Design review of the part built by this model. Coordinates are the model's own, in mm. Face numbers are marked on the shaded views. A direction names the side the tool comes from. Give positions to 0.01 mm unless a question says otherwise; leave off trailing zeros. Write each loop counter-clockwise with the first axis right and the second up, starting at its lowest first coordinate (ties: lowest second). Pieces come first, ordered by that corner, then holes. Notation, with made-up numbers: (17, 3.25) -> (38, 3.25) arc R6 cw to (38, 10.25) -> close; hole circle Ø5 at (47.25, 47). An arc over 180 degrees is marked (long way). Answer as a JSON object with one key per item and string values.
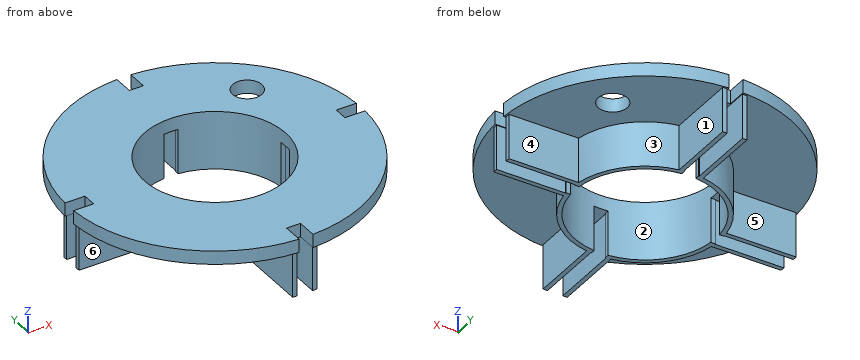
```python
from build123d import *

# Parameters (mm, degrees)
CYLINDER_R     = 3.25
CYLINDER_DEPTH = 10
BOX030_W       = 3
BOX030_H       = 3
BOX030_DEPTH   = 3
BOX047_W       = 3
BOX047_H       = 3
BOX047_DEPTH   = 3
BOX029_W       = 3
BOX029_H       = 3
BOX029_DEPTH   = 3
BOX028_W       = 3
BOX028_H       = 3
BOX028_DEPTH   = 3
BOX043_W       = 3.1
BOX043_H       = 6
BOX043_DEPTH   = 10
BOX044_W       = 3.1
BOX044_H       = 6
BOX044_DEPTH   = 10
BOX045_W       = 6
BOX045_H       = 3.1
BOX045_DEPTH   = 10
BOX046_W       = 6
BOX046_H       = 3.1
BOX046_DEPTH   = 10
BOX032_W       = 3.1
BOX032_H       = 6
BOX032_DEPTH   = 3
BOX033_W       = 6
BOX033_H       = 3.1
BOX033_DEPTH   = 3
BOX034_W       = 6
BOX034_H       = 3.1
BOX034_DEPTH   = 3
BOX031_W       = 3.1
BOX031_H       = 6
BOX031_DEPTH   = 3
TUBE003_R      = 16.7
TUBE003_R_2    = 15.7
TUBE003_DEPTH  = 10
BOX036_W       = 1
BOX036_H       = 16
BOX036_DEPTH   = 10
BOX037_W       = 1
BOX037_H       = 16
BOX037_DEPTH   = 10
BOX038_W       = 1
BOX038_H       = 16
BOX038_DEPTH   = 10
BOX039_W       = 16
BOX039_H       = 1
BOX039_DEPTH   = 10
BOX040_W       = 16
BOX040_H       = 1
BOX040_DEPTH   = 10
BOX041_W       = 16
BOX041_H       = 1
BOX041_DEPTH   = 10
BOX042_W       = 16
BOX042_H       = 1
BOX042_DEPTH   = 10
BOX035_W       = 1
BOX035_H       = 16
BOX035_DEPTH   = 10
TUBE002_R      = 32.5
TUBE002_R_2    = 15.7
TUBE002_DEPTH  = 3


with BuildPart() as eyeboltcutout:
    # Cylinder → Cylinder (new body)
    with BuildSketch(Plane(origin=(17.5, 16.5, 91), x_dir=(1, 0, 0), z_dir=(0, 0, 1))):
        Circle(CYLINDER_R)
    extrude(amount=CYLINDER_DEPTH)


with BuildPart() as finlock015:
    # Box030 → Box030 (new body)
    with BuildSketch(Plane(origin=(-1.5, 21, -3), x_dir=(1, 0, 0), z_dir=(0, 0, 1))):
        with Locations((1.5, 1.5)):
            Rectangle(BOX030_W, BOX030_H)
    extrude(amount=BOX030_DEPTH)


with BuildPart() as finlock016:
    # Box047 → Box047 (new body)
    with BuildSketch(Plane(origin=(-1.5, -24, -3), x_dir=(1, 0, 0), z_dir=(0, 0, 1))):
        with Locations((1.5, 1.5)):
            Rectangle(BOX047_W, BOX047_H)
    extrude(amount=BOX047_DEPTH)


with BuildPart() as finlock014:
    # Box029 → Box029 (new body)
    with BuildSketch(Plane(origin=(-24, -1.5, -3), x_dir=(1, 0, 0), z_dir=(0, 0, 1))):
        with Locations((1.5, 1.5)):
            Rectangle(BOX029_W, BOX029_H)
    extrude(amount=BOX029_DEPTH)


with BuildPart() as finlocks001:
    # Box028 → Box028 (new body)
    with BuildSketch(Plane(origin=(21, -1.5, -3), x_dir=(1, 0, 0), z_dir=(0, 0, 1))):
        with Locations((1.5, 1.5)):
            Rectangle(BOX028_W, BOX028_H)
    extrude(amount=BOX028_DEPTH)

    # Fusion014: union FinLock015, FinLock016, FinLock014
    add(finlock015.part)
    add(finlock016.part)
    add(finlock014.part)


with BuildPart() as fincut013:
    # Box043 → Box043 (new body)
    with BuildSketch(Plane(origin=(-1.55, -21, -10), x_dir=(1, 0, 0), z_dir=(0, 0, 1))):
        with Locations((1.55, 3)):
            Rectangle(BOX043_W, BOX043_H)
    extrude(amount=BOX043_DEPTH)


with BuildPart() as fincut014:
    # Box044 → Box044 (new body)
    with BuildSketch(Plane(origin=(-1.55, 15, -10), x_dir=(1, 0, 0), z_dir=(0, 0, 1))):
        with Locations((1.55, 3)):
            Rectangle(BOX044_W, BOX044_H)
    extrude(amount=BOX044_DEPTH)


with BuildPart() as fincut015:
    # Box045 → Box045 (new body)
    with BuildSketch(Plane(origin=(15, -1.55, -10), x_dir=(1, 0, 0), z_dir=(0, 0, 1))):
        with Locations((3, 1.55)):
            Rectangle(BOX045_W, BOX045_H)
    extrude(amount=BOX045_DEPTH)


with BuildPart() as innerfincutouts001:
    # Box046 → Box046 (new body)
    with BuildSketch(Plane(origin=(-21, -1.55, -10), x_dir=(1, 0, 0), z_dir=(0, 0, 1))):
        with Locations((3, 1.55)):
            Rectangle(BOX046_W, BOX046_H)
    extrude(amount=BOX046_DEPTH)

    # Fusion011: union FinCut013, FinCut014, FinCut015
    add(fincut013.part)
    add(fincut014.part)
    add(fincut015.part)


with BuildPart() as fincut010:
    # Box032 → Box032 (new body)
    with BuildSketch(Plane(origin=(-1.55, 28, 0), x_dir=(1, 0, 0), z_dir=(0, 0, 1))):
        with Locations((1.55, 3)):
            Rectangle(BOX032_W, BOX032_H)
    extrude(amount=BOX032_DEPTH)


with BuildPart() as fincut011:
    # Box033 → Box033 (new body)
    with BuildSketch(Plane(origin=(28, -1.55, 0), x_dir=(1, 0, 0), z_dir=(0, 0, 1))):
        with Locations((3, 1.55)):
            Rectangle(BOX033_W, BOX033_H)
    extrude(amount=BOX033_DEPTH)


with BuildPart() as fincut012:
    # Box034 → Box034 (new body)
    with BuildSketch(Plane(origin=(-34, -1.55, 0), x_dir=(1, 0, 0), z_dir=(0, 0, 1))):
        with Locations((3, 1.55)):
            Rectangle(BOX034_W, BOX034_H)
    extrude(amount=BOX034_DEPTH)


with BuildPart() as fincutouts001:
    # Box031 → Box031 (new body)
    with BuildSketch(Plane(origin=(-1.55, -34, 0), x_dir=(1, 0, 0), z_dir=(0, 0, 1))):
        with Locations((1.55, 3)):
            Rectangle(BOX031_W, BOX031_H)
    extrude(amount=BOX031_DEPTH)

    # Fusion009: union FinCut010, FinCut011, FinCut012
    add(fincut010.part)
    add(fincut011.part)
    add(fincut012.part)

    # Fusion012: union InnerFinCutouts001
    add(innerfincutouts001.part)


with BuildPart() as innertube001:
    # Tube003 → Tube003 (new body)
    with BuildSketch(Plane.XY.offset(-10)):
        Circle(TUBE003_R)
        Circle(TUBE003_R_2, mode=Mode.SUBTRACT)
    extrude(amount=TUBE003_DEPTH)


with BuildPart() as alignment010:
    # Box036 → Box036 (new body)
    with BuildSketch(Plane(origin=(-2.7, 16, -10), x_dir=(1, 0, 0), z_dir=(0, 0, 1))):
        with Locations((0.5, 8)):
            Rectangle(BOX036_W, BOX036_H)
    extrude(amount=BOX036_DEPTH)


with BuildPart() as alignment011:
    # Box037 → Box037 (new body)
    with BuildSketch(Plane(origin=(-2.7, -32, -10), x_dir=(1, 0, 0), z_dir=(0, 0, 1))):
        with Locations((0.5, 8)):
            Rectangle(BOX037_W, BOX037_H)
    extrude(amount=BOX037_DEPTH)


with BuildPart() as alignment012:
    # Box038 → Box038 (new body)
    with BuildSketch(Plane(origin=(1.7, -32, -10), x_dir=(1, 0, 0), z_dir=(0, 0, 1))):
        with Locations((0.5, 8)):
            Rectangle(BOX038_W, BOX038_H)
    extrude(amount=BOX038_DEPTH)


with BuildPart() as alignment013:
    # Box039 → Box039 (new body)
    with BuildSketch(Plane(origin=(16, 1.7, -10), x_dir=(1, 0, 0), z_dir=(0, 0, 1))):
        with Locations((8, 0.5)):
            Rectangle(BOX039_W, BOX039_H)
    extrude(amount=BOX039_DEPTH)


with BuildPart() as alignment014:
    # Box040 → Box040 (new body)
    with BuildSketch(Plane(origin=(16, -2.7, -10), x_dir=(1, 0, 0), z_dir=(0, 0, 1))):
        with Locations((8, 0.5)):
            Rectangle(BOX040_W, BOX040_H)
    extrude(amount=BOX040_DEPTH)


with BuildPart() as alignment015:
    # Box041 → Box041 (new body)
    with BuildSketch(Plane(origin=(-32, 1.7, -10), x_dir=(1, 0, 0), z_dir=(0, 0, 1))):
        with Locations((8, 0.5)):
            Rectangle(BOX041_W, BOX041_H)
    extrude(amount=BOX041_DEPTH)


with BuildPart() as alignment016:
    # Box042 → Box042 (new body)
    with BuildSketch(Plane(origin=(-32, -2.7, -10), x_dir=(1, 0, 0), z_dir=(0, 0, 1))):
        with Locations((8, 0.5)):
            Rectangle(BOX042_W, BOX042_H)
    extrude(amount=BOX042_DEPTH)


with BuildPart() as alignmenttabs001:
    # Box035 → Box035 (new body)
    with BuildSketch(Plane(origin=(1.7, 16, -10), x_dir=(1, 0, 0), z_dir=(0, 0, 1))):
        with Locations((0.5, 8)):
            Rectangle(BOX035_W, BOX035_H)
    extrude(amount=BOX035_DEPTH)

    # Fusion010: union Alignment010, Alignment011, Alignment012, Alignment013, Alignment014, Alignment015, Alignment016
    add(alignment010.part)
    add(alignment011.part)
    add(alignment012.part)
    add(alignment013.part)
    add(alignment014.part)
    add(alignment015.part)
    add(alignment016.part)


with BuildPart() as cut004:
    # Tube002 → Tube002 (new body)
    with BuildSketch(Plane.XY):
        Circle(TUBE002_R)
        Circle(TUBE002_R_2, mode=Mode.SUBTRACT)
    extrude(amount=TUBE002_DEPTH)

    # Fusion013: union InnerTube001, AlignmentTabs001
    add(innertube001.part)
    add(alignmenttabs001.part)

    # Cut003: cut FinCutouts001
    add(fincutouts001.part, mode=Mode.SUBTRACT)

    # Connect001: union FinLocks001
    add(finlocks001.part)


with BuildPart() as cut004_1:
    # Connect001 placement: moved
    add(cut004.part.moved(Location((0, 0, 95))))

    # Cut004: cut EyeboltCutout
    add(eyeboltcutout.part, mode=Mode.SUBTRACT)


solid = cut004_1.part
```
(1) For line 1 along X through (y, z) = (16.5, 97.45); line 2 along Y through (x, z) = (28.5, 95.25); line 3 along X through (y, z) = (-21, 90), list the stretches that pass through material, from the lowest coordinate up.
Here are the results:
{"line 1": "x = -28 to 14.25, 20.75 to 28", "line 2": "y = -15.62 to -1.55, 1.55 to 15.62", "line 3": "x = -2.7 to -1.7, 1.7 to 2.7"}
(2) We need section A-A, the plane x = 0. State the section outline as (y, z) points.
Here are the results:
{"outline": "(-28, 95) -> (-24, 95) -> (-24, 92) -> (-21, 92) -> (-21, 95) -> (-15.7, 95) -> (-15.7, 98) -> (-28, 98) -> close; (15.7, 95) -> (21, 95) -> (21, 92) -> (24, 92) -> (24, 95) -> (28, 95) -> (28, 98) -> (15.7, 98) -> close"}
(3) Clearance check with flat-ended pins moving along their axes: pin 1 (3.5 mm diameter, centred on y = -22.5, z = 93.5, fed in from +X); pin 2 (5 mm diameter, centred on y = 24, z = 87, fed in from -X); pin 3 (3.5 mm diameter, centred on y = -0.5, z = 93, fed in from +X). State where each tip first meets the part, or that it passes through.
Here are the results:
{"pin 1": "stops at x = 24.28", "pin 2": "stops at x = -2.7", "pin 3": "stops at x = 32"}
(4) The part is to be moulded in two halves that separate along Y. For the marked faces 1, 2 and 3, say which applies: +Y half, -Y half, draft (parallel to the pull), parting line (faces both ways), or undercut.
Here are the results:
{"face 1": "draft", "face 2": "undercut", "face 3": "+Y half"}
(5) We need section D-D, the plane y = -26. State the section outline as (x, z) points, then the cut area to 3 significant figures.
Here are the results:
{"outline": "(-19.5, 95) -> (-2.7, 95) -> (-2.7, 85) -> (-1.7, 85) -> (-1.7, 95) -> (1.7, 95) -> (1.7, 85) -> (2.7, 85) -> (2.7, 95) -> (19.5, 95) -> (19.5, 98) -> (-19.5, 98) -> close", "area": "137 mm²"}
(6) We need section C-C, the plane z = 89.5. Give the number of separate pieces and of enclosed holes in the cut face, then the cut area to 3 significant figures.
Here are the results:
{"separate pieces": "4", "enclosed holes": "0", "area": "213 mm²"}
(7) For the marked faces 4, 5 and 6, list the 3-axis set-ups (+Z, -Z, +X, -X, +Y, -Y) from which the entire face can be reached by the end or side of a thin tool; tool diameter is ignored.
Here are the results:
{"face 4": "-Z, +X, +Y", "face 5": "-Z, -X, +Y", "face 6": "-Z, -X, -Y"}
